from build123d import *

# Parameters (mm, degrees)
SKETCH1_W            = 73
SKETCH1_H            = 40
BOSS_EXTRUDE1_DEPTH  = 5
SKETCH2_W            = 92
SKETCH2_H            = 40
BOSS_EXTRUDE2_DEPTH  = 3
M3_CLEARANCE_HOLE1_D = 3.6
M3_CLEARANCE_HOLE2_D = 3.4
SKETCH9_R            = 11
CUT_EXTRUDE1_DEPTH   = 9


with BuildPart() as part:
    # Sketch1 → Boss-Extrude1 (new body)
    with BuildSketch(Plane(origin=(0, 0, 0), x_dir=(1, 0, 0), z_dir=(0, 1, 0))):
        Rectangle(SKETCH1_W, SKETCH1_H)
    extrude(amount=BOSS_EXTRUDE1_DEPTH)

    # Sketch2 → Boss-Extrude2 (add)
    with BuildSketch(Plane.XZ):
        Rectangle(SKETCH2_W, SKETCH2_H)
    extrude(amount=BOSS_EXTRUDE2_DEPTH)

    # M3 Clearance Hole1 (through all)
    with Locations(Plane(origin=(0, 0, 0), x_dir=(1, 0, 0), z_dir=(0, 1, 0))):
        with Locations((-40.5, 15.25), (-40.5, -15.25), (40.5, 15.25), (40.5, -15.25)):
            Hole(M3_CLEARANCE_HOLE1_D / 2)

    # M3 Clearance Hole2 (through all)
    with Locations(Plane(origin=(0, 5, 0), x_dir=(1, 0, 0), z_dir=(0, 1, 0))):
        with Locations((0, 0), (15.25, 15.25), (-15.25, -15.25), (-15.25, 15.25), (15.25, -15.25)):
            Hole(M3_CLEARANCE_HOLE2_D / 2)

    # Sketch9 → Cut-Extrude1 (cut, through all)
    with BuildSketch(Plane(origin=(0, 5, 0), x_dir=(1, 0, 0), z_dir=(0, 1, 0))):
        Circle(SKETCH9_R)
    extrude(amount=-CUT_EXTRUDE1_DEPTH, mode=Mode.SUBTRACT)


solid = part.part
Part model, mm, in its own coordinate system. A direction names the side the tool comes from. Round coordinates to 2 decimals unless told otherwise and drop trailing zeros. Write each loop counter-clockwise with the first axis right and the second up, starting at its lowest first coordinate (ties: lowest second). Pieces come first, ordered by that corner, then holes. Notation, with made-up numbers: M 52,-10.5 L 60,-10.5 A17 ccw 60,0.5 Z; hole C -30.5,56.5 d9. An arc over 180 degrees is marked long. Return JSON: item names as keys, results as strings. Group by question number.
(1) Drill centre lines: probe 1 along Z at (x, y) = (40.5, -2.15); probe 2 along X at (y, z) = (3.25, -15.25); probe 3 along X at (y, z) = (-0.9, 15.25). Where is each one in solid material? Low to high.
(2) Saw through at A-A on x = -40.5. Write the cut outline in (y, z), then the cut area to 3 significant figures.
(3) Two-plate mould, pull along X, no slides. Class faces 1 (the face through (39.532, -1.521, 13.732)), 2 (the face through (46, -1, 0)), 3 (the face through (-41, 0, 0)): +X half, -X half, draft (parallel to the pull), parting line (faces both ways), or undercut.
(4) Saw through at C-C on y = 2.5. Write the cut outline in (x, z), then the cut area to 3 significant figures.
(5) Pin check, flat tips, straight feed: pin 1 Ø2 at (y, z) = (3, 10.5) entering from -X; pin 2 Ø5 at (x, z) = (41.5, -9.5) entering from +Y; pin 3 Ø1.5 at (y, z) = (1.5, -3.5) entering from +X. Stop position of each tip, or through.
(6) Saw through at D-D on x = 0. Write the cut outline in (y, z), then the cut area to 3 significant figures.
(7) Which spindle directions (+Z, -Z, +X, -X, +Y, -Y) get a long thin tool onto all of the face, cutting with end or side? Do faces 4 (the face through (41, 0, 0)), 5 (the face through (-46, -1, 0)), 6 (the face through (-36.5, 2, 0)). Say none if no direction does.
(8) Saw through at B-B on z = -15.25. Write the cut outline in (x, y).
Returned:
{
 "1": {"probe 1": "-20 to -17.05, -13.45 to 13.45, 17.05 to 20", "probe 2": "-36.5 to -16.95, -13.55 to 13.55, 16.95 to 36.5", "probe 3": "-46 to -42.3, -38.7 to -16.95, -13.55 to 13.55, 16.95 to 38.7, 42.3 to 46"},
 "2": {"outline": "M -3,-20 L 0,-20 L 0,-17.05 L -3,-17.05 Z; M -3,-13.45 L 0,-13.45 L 0,13.45 L -3,13.45 Z; M -3,17.05 L 0,17.05 L 0,20 L -3,20 Z", "area": "98.4 mm²"},
 "3": {"face 1": "undercut", "face 2": "+X half", "face 3": "draft"},
 "4": {"outline": "M -36.5,-20 L 36.5,-20 L 36.5,20 L -36.5,20 Z; hole C -15.25,-15.25 d3.4; hole C -15.25,15.25 d3.4; hole C 0,0 d22; hole C 15.25,-15.25 d3.4; hole C 15.25,15.25 d3.4", "area": "2,500 mm²"},
 "5": {"pin 1": "x = -36.5", "pin 2": "y = 0", "pin 3": "x = 36.5"},
 "6": {"outline": "M -3,-20 L 5,-20 L 5,-11 L -3,-11 Z; M -3,11 L 5,11 L 5,20 L -3,20 Z", "area": "144 mm²"},
 "7": {"face 4": "+Z, -Z, +X, +Y", "face 5": "+Z, -Z, -X, +Y, -Y", "face 6": "+Z, -Z, -X, +Y"},
 "8": {"outline": "M -46,-3 L -42.3,-3 L -42.3,0 L -46,0 Z; M -38.7,-3 L -16.95,-3 L -16.95,5 L -36.5,5 L -36.5,0 L -38.7,0 Z; M -13.55,-3 L 13.55,-3 L 13.55,5 L -13.55,5 Z; M 16.95,-3 L 38.7,-3 L 38.7,0 L 36.5,0 L 36.5,5 L 16.95,5 Z; M 42.3,-3 L 46,-3 L 46,0 L 42.3,0 Z"}
}
